```python
from build123d import *

# Parameters (mm, degrees)
SKETCH_1_W          = 260
SKETCH_1_H          = 55
EXTRUDE_1_DEPTH     = 3
FILLET_1_R          = 2
SKETCH_2_R          = 1.6
CUT_EXTRUDE_1_DEPTH = 18
CUT_EXTRUDE_2_DEPTH = 10


with BuildPart() as part:
    # 草图1 → 凸台-拉伸1 (new body)
    with BuildSketch(Plane.XY):
        Rectangle(SKETCH_1_W, SKETCH_1_H)
    extrude(amount=EXTRUDE_1_DEPTH)

    # 圆角1
    fillet_1_edges = [part.edges().sort_by_distance(p)[0] for p in [
        (-130, 27.5, 1.5),
        (130, 27.5, 1.5),
        (130, -27.5, 1.5),
        (-130, -27.5, 1.5),
    ]]
    fillet(fillet_1_edges, radius=FILLET_1_R)

    # 草图2 → 切除-拉伸1 (cut)
    with BuildSketch(Plane.XY.offset(3)):
        with Locations((-122, 17.5)):
            Circle(SKETCH_2_R)
        with Locations((-122, -2.5)):
            Circle(SKETCH_2_R)
        with Locations((122, -2.5)):
            Circle(SKETCH_2_R)
        with Locations((122, 17.5)):
            Circle(SKETCH_2_R)
    extrude(amount=-CUT_EXTRUDE_1_DEPTH, mode=Mode.SUBTRACT)

    # 草图3 → 切除-拉伸2 (cut)
    with BuildSketch(Plane.XY.offset(3)):
        with BuildLine():
            Line((-106, 20), (-106, -20))
            ThreePointArc((-106, -20), (-109, -23), (-112, -20))
            Line((-112, -20), (-112, 20))
            ThreePointArc((-112, 20), (-109, 23), (-106, 20))
        make_face()
        with BuildLine():
            Line((-96, 20), (-96, -20))
            ThreePointArc((-96, -20), (-99, -23), (-102, -20))
            Line((-102, -20), (-102, 20))
            ThreePointArc((-102, 20), (-99, 23), (-96, 20))
        make_face()
        with BuildLine():
            Line((-86, 20), (-86, -20))
            ThreePointArc((-86, -20), (-89, -23), (-92, -20))
            Line((-92, -20), (-92, 20))
            ThreePointArc((-92, 20), (-89, 23), (-86, 20))
        make_face()
        with BuildLine():
            Line((-76, 20), (-76, -20))
            ThreePointArc((-76, -20), (-79, -23), (-82, -20))
            Line((-82, -20), (-82, 20))
            ThreePointArc((-82, 20), (-79, 23), (-76, 20))
        make_face()
        with BuildLine():
            Line((-66, 20), (-66, -20))
            ThreePointArc((-66, -20), (-69, -23), (-72, -20))
            Line((-72, -20), (-72, 20))
            ThreePointArc((-72, 20), (-69, 23), (-66, 20))
        make_face()
        with BuildLine():
            Line((-56, 20), (-56, -20))
            ThreePointArc((-56, -20), (-59, -23), (-62, -20))
            Line((-62, -20), (-62, 20))
            ThreePointArc((-62, 20), (-59, 23), (-56, 20))
        make_face()
        with BuildLine():
            Line((-46, 20), (-46, -20))
            ThreePointArc((-46, -20), (-49, -23), (-52, -20))
            Line((-52, -20), (-52, 20))
            ThreePointArc((-52, 20), (-49, 23), (-46, 20))
        make_face()
        with BuildLine():
            Line((-36, 20), (-36, -20))
            ThreePointArc((-36, -20), (-39, -23), (-42, -20))
            Line((-42, -20), (-42, 20))
            ThreePointArc((-42, 20), (-39, 23), (-36, 20))
        make_face()
        with BuildLine():
            Line((-26, 20), (-26, -20))
            ThreePointArc((-26, -20), (-29, -23), (-32, -20))
            Line((-32, -20), (-32, 20))
            ThreePointArc((-32, 20), (-29, 23), (-26, 20))
        make_face()
        with BuildLine():
            Line((-16, 20), (-16, -20))
            ThreePointArc((-16, -20), (-19, -23), (-22, -20))
            Line((-22, -20), (-22, 20))
            ThreePointArc((-22, 20), (-19, 23), (-16, 20))
        make_face()
        with BuildLine():
            Line((-6, 20), (-6, -20))
            ThreePointArc((-6, -20), (-9, -23), (-12, -20))
            Line((-12, -20), (-12, 20))
            ThreePointArc((-12, 20), (-9, 23), (-6, 20))
        make_face()
        with BuildLine():
            Line((4, 20), (4, -20))
            ThreePointArc((4, -20), (1, -23), (-2, -20))
            Line((-2, -20), (-2, 20))
            ThreePointArc((-2, 20), (1, 23), (4, 20))
        make_face()
        with BuildLine():
            Line((14, 20), (14, -20))
            ThreePointArc((14, -20), (11, -23), (8, -20))
            Line((8, -20), (8, 20))
            ThreePointArc((8, 20), (11, 23), (14, 20))
        make_face()
        with BuildLine():
            Line((24, 20), (24, -20))
            ThreePointArc((24, -20), (21, -23), (18, -20))
            Line((18, -20), (18, 20))
            ThreePointArc((18, 20), (21, 23), (24, 20))
        make_face()
        with BuildLine():
            Line((34, 20), (34, -20))
            ThreePointArc((34, -20), (31, -23), (28, -20))
            Line((28, -20), (28, 20))
            ThreePointArc((28, 20), (31, 23), (34, 20))
        make_face()
        with BuildLine():
            Line((44, 20), (44, -20))
            ThreePointArc((44, -20), (41, -23), (38, -20))
            Line((38, -20), (38, 20))
            ThreePointArc((38, 20), (41, 23), (44, 20))
        make_face()
        with BuildLine():
            Line((54, 20), (54, -20))
            ThreePointArc((54, -20), (51, -23), (48, -20))
            Line((48, -20), (48, 20))
            ThreePointArc((48, 20), (51, 23), (54, 20))
        make_face()
        with BuildLine():
            Line((64, 20), (64, -20))
            ThreePointArc((64, -20), (61, -23), (58, -20))
            Line((58, -20), (58, 20))
            ThreePointArc((58, 20), (61, 23), (64, 20))
        make_face()
        with BuildLine():
            Line((74, 20), (74, -20))
            ThreePointArc((74, -20), (71, -23), (68, -20))
            Line((68, -20), (68, 20))
            ThreePointArc((68, 20), (71, 23), (74, 20))
        make_face()
        with BuildLine():
            Line((84, 20), (84, -20))
            ThreePointArc((84, -20), (81, -23), (78, -20))
            Line((78, -20), (78, 20))
            ThreePointArc((78, 20), (81, 23), (84, 20))
        make_face()
        with BuildLine():
            Line((94, 20), (94, -20))
            ThreePointArc((94, -20), (91, -23), (88, -20))
            Line((88, -20), (88, 20))
            ThreePointArc((88, 20), (91, 23), (94, 20))
        make_face()
        with BuildLine():
            Line((104, 20), (104, -20))
            ThreePointArc((104, -20), (101, -23), (98, -20))
            Line((98, -20), (98, 20))
            ThreePointArc((98, 20), (101, 23), (104, 20))
        make_face()
        with BuildLine():
            Line((114, 20), (114, -20))
            ThreePointArc((114, -20), (111, -23), (108, -20))
            Line((108, -20), (108, 20))
            ThreePointArc((108, 20), (111, 23), (114, 20))
        make_face()
    extrude(amount=-CUT_EXTRUDE_2_DEPTH, mode=Mode.SUBTRACT)


solid = part.part
```
The listing builds one solid part. Answer for the finished solid, in the listing's coordinates (mm). Round coordinates to 2 decimals unless told otherwise and drop trailing zeros. Loops run counter-clockwise (first coordinate to the right, second up) from the corner with the lowest first, then second, coordinate; pieces in that order, holes last.
Q1. Section A-A, the plane x = 11 is taken. Determine the outline of the cut face in (y, z), then the cut area to 3 significant figures.
Q2. Section B-B, the plane z = 2.5 is taken. Count the separate pieces of the cut face and the enclosed holes in it, then the cut area to 3 significant figures.
Q3. Given pin 1 Ø2.5 at (x, y) = (-122, 17.5) entering from +Z, flat-ended and moving along its own axis, determine where the tip first touches the part or whether it passes through.
Q4. Find the intervals of material crossed by line 1 (Y direction, x = 122, z = 1.85); line 2 (Y direction, x = -9, z = 1.15); line 3 (Y direction, x = -1, z = 2), in increasing order.
Completed:
1. outline: (-27.5, 0) - (-23, 0) - (-23, 3) - (-27.5, 3) - close; (23, 0) - (27.5, 0) - (27.5, 3) - (23, 3) - close
1. area: 27.0 mm2
2. separate pieces: 1
2. enclosed holes: 27
2. area: 8,090 mm2
3. pin 1: passes through
4. line 1: y = -27.5 to -4.1, -0.9 to 15.9, 19.1 to 27.5
4. line 2: y = -27.5 to -23, 23 to 27.5
4. line 3: y = -27.5 to -22.24, 22.24 to 27.5
